Model file for the job. Use its own axes, mm. A direction names the side the tool comes from. Give positions to 0.01 mm unless a question says otherwise; leave off trailing zeros. Loops run counter-clockwise (first coordinate to the right, second up) from the corner with the lowest first, then second, coordinate; pieces in that order, holes last. Notation, with made-up numbers: (48.5, -13) -> (70.5, -13) arc R20 cw to (70.5, 20) -> close; hole circle Ø10 at (77.5, -24.5). An arc over 180 degrees is marked (long way). Use CSV: the item, a comma, the result in double quotes. Start each with the question number.
(1) Flat gauge pins, fed straight in: pin 1 (0.6 mm diameter, centred on y = 9, z = 2, fed in from +X); pin 2 (1.6 mm diameter, centred on y = 14.5, z = 1, fed in from -X); pin 3 (0.9 mm diameter, centred on y = 12, z = 2, fed in from +X). Where does each tip first touch, or does it go through?
(2) 3-axis set-ups, long thin cutter, end or side, ignore diameter. For faces 4 (the flat face through (4.255, 14, 1)), 5 (the flat face through (5, 11.124, 1)), 6 (the flat face through (2.646, 10, 1)), 7 (the flat face through (1.128, 16, -4)), 8 (the cylindrical face through (-5.7, 4.7, -2)): which of +Z, -Z, +X, -X, +Y, -Y reach the whole face in a straight line?
(3) Cut at B-B on x = -2.25. Write the cut outline in (y, z).
(4) Cut at C-C on x = 8. Write the cut outline in (y, z).
(5) Cut at A-A on y = 16. State how many separate pieces and enclosed holes the cut face has, then the cut area to 3 significant figures.
(6) Pull direction X, two halves, no side cores. Call faces 1 (the flat face through (-0.14, 22.86, 1.48)), 2 (the flat face through (-3, 10, -1)), 3 (the flat face through (3.12, 7.43, 1.48)): pulls with the +X half, pulls with the -X half, needs draft (parallel to the pull), parting line crosses it, or undercut.
(7) Cut at D-D on y = 22. Write the cut outline in (x, z), then the cut area to 3 significant figures.
(8) Drill centre lines: probe 1 along X at (y, z) = (2, -3); probe 2 along X at (y, z) = (3, -2.75); probe 3 along Z at (x, y) = (4.75, -0.5). Where is each one in solid material? Low to high.
from build123d import *

# Parameters (mm, degrees)
BOSS_SWITCH_BODY_DEPTH                    = 3
SKETCH1_W                                 = 4.0875
SKETCH1_H                                 = 1.5
SKETCH1_W_2                               = 3.046903414
SKETCH1_H_2                               = 3.5
BOSS_FLANGE_WIDTH_DEPTH                   = 5
SKETCH2_W                                 = 4
SKETCH2_H                                 = 2
SKETCH2_W_2                               = 8
SKETCH2_H_2                               = 1.5
BOSS_FLANGE_HEIGHT_DEPTH                  = 10.620596586
CUT_UP_TO_DOWN_DERAILLEUR_CLEARANCE_REACH = 23.629
SKETCH10_W                                = 1.5
SKETCH10_H                                = 3
SKETCH17_W                                = 12.1675
SKETCH17_H                                = 4
BOSS_FLANGE_SUPPORT_DEPTH                 = 17.508325141
TAP_DRILL_FOR_M2X0_4_TAP1_D               = 1.6
M2_CLEARANCE_HOLE2_D                      = 2.4
M2_CLEARANCE_HOLE2_DEPTH                  = 15
M2_CLEARANCE_HOLE2_TIP                    = 0.721032743
CHAMFER_FLANGE_SUPPORT_SIZE               = 1.5
CHAMFER_FLANGE_SUPPORT_2_SIZE             = 1.5
SKETCH23_W                                = 7.349718646
SKETCH23_H                                = 15.508325141
CUT_GAP_FOR_PRINTING_DEPTH                = 32.000499688
CUT_WIDE_DERAILLEUR_CLEARANCE_DEPTH       = 33.195879702
CUT_WIDE_DERAILLEUR_CLEARANCE_DEPTH_BACK  = 4
SKETCH27_W                                = 2.5
SKETCH27_H                                = 3.5
CHAMFER9_SIZE                             = 1.25
SKETCH28_W                                = 3.046903414
SKETCH28_H                                = 1
CUT_EXTRUDE1_DEPTH                        = 1
CHAMFER10_SIZE                            = 0.5
CHAMFER_FLANGE_SUPPORT_3_SIZE             = 1
CUT_EXTRUDE2_DEPTH                        = 34.862828732
BOSS_EXTRUDE2_DEPTH                       = 8.2


with BuildPart() as part:
    # Sketch-SwitchBossUp → Boss-Switch Body (new body)
    with BuildSketch(Plane.XY):
        with BuildLine():
            Line((5.581091204, 12.554885442), (5.58109997, 11.370542897))
            Line((5.58109997, 11.370542897), (5.154266051, 11.12411022))
            Line((5.154266051, 11.12411022), (3.971266051, 11.12411022))
            Line((3.971266051, 11.12411022), (3.97126394, 11.79911022))
            Line((3.97126394, 11.79911022), (3.296271341, 11.409403061))
            Line((3.296271341, 11.409403061), (3.296271341, 9.409403061))
            Line((3.296271341, 9.409403061), (3.971278743, 9.019687356))
            Line((3.971278743, 9.019687356), (3.971278743, 9.409408058))
            Line((3.971278743, 9.409408058), (5.333511297, 10.40941814))
            Line((5.333511297, 10.40941814), (6.133511297, 10.409424062))
            Line((6.133511297, 10.409424062), (6.627976927, 9.860264345))
            Line((6.627976927, 9.860264345), (6.627976927, 8.007577878))
            Line((6.627976927, 8.007577878), (6.081127833, 7.606137899))
            Line((6.081127833, 7.606137899), (5.581127833, 7.606137899))
            Line((5.581127833, 7.606137899), (4.906138119, 7.216432406))
            Line((4.906138119, 7.216432406), (4.906138119, 5.216432406))
            Line((4.906138119, 5.216432406), (5.58114552, 4.826716701))
            Line((5.58114552, 4.826716701), (6.290476927, 4.826716701))
            Line((6.290476927, 4.826716701), (6.290476927, 3.076720436))
            Line((6.290476927, 3.076720436), (5.040476927, 1.826720436))
            Line((5.040476927, 1.826720436), (5.040476927, -0.673279564))
            Line((5.040476927, -0.673279564), (6.627976927, -0.673279564))
            Line((6.627976927, -0.673279564), (6.627976927, -3.673279564))
            Line((6.627976927, -3.673279564), (2.540476927, -3.673279564))
            Line((2.540476927, -3.673279564), (2.540476927, -2.173279564))
            Line((2.540476927, -2.173279564), (4.040476927, -0.673279564))
            Line((4.040476927, -0.673279564), (4.040476927, 1.826720436))
            Line((4.040476927, 1.826720436), (2.790476927, 3.076720436))
            Line((2.790476927, 3.076720436), (2.790476927, 4.826720436))
            Line((2.790476927, 4.826720436), (3.58114552, 4.826720436))
            Line((3.58114552, 4.826720436), (4.256138119, 5.216427595))
            Line((4.256138119, 5.216427595), (4.256138119, 7.216427595))
            Line((4.256138119, 7.216427595), (3.581130717, 7.6061433))
            Line((3.581130717, 7.6061433), (2.64686251, 7.249572244))
            Line((2.64686251, 7.249572244), (1.971281627, 9.019692757))
            Line((1.971281627, 9.019692757), (2.646271341, 9.40939825))
            Line((2.646271341, 9.40939825), (2.646271341, 11.40939825))
            Line((2.646271341, 11.40939825), (1.696557212, 11.957715958))
            Line((1.696557212, 11.957715958), (0.573317845, 12.60621851))
            Line((0.573317845, 12.60621851), (-0.645153605, 19.844362607))
            ThreePointArc((-0.645153605, 19.844362607), (-0.473707256, 20.590279886), (0.174966786, 20.996492176))
            Line((0.174966786, 20.996492176), (-0.46073685, 24.772792819))
            ThreePointArc((-0.46073685, 24.772792819), (-1.019582136, 24.919522879), (-1.541303694, 25.167805745))
            ThreePointArc((-1.541303694, 25.167805745), (-2.872284003, 26.795385437), (-2.852546321, 28.897797067))
            ThreePointArc((-2.852546321, 28.897797067), (-1.887813913, 29.338582026), (-1.447028953, 28.373849618))
            ThreePointArc((-1.447028953, 28.373849618), (-0.703448682, 26.416936722), (1.333779254, 26.898727173))
            ThreePointArc((1.333779254, 26.898727173), (2.379722745, 27.074801628), (2.555797201, 26.028858137))
            ThreePointArc((2.555797201, 26.028858137), (2.086504637, 25.507104397), (1.511513111, 25.104801997))
            Line((1.511513111, 25.104801997), (1.553598189, 24.854801997))
            Line((1.553598189, 24.854801997), (9.027976927, 24.854801997))
            Line((9.027976927, 24.854801997), (9.027976927, 22.354801997))
            Line((9.027976927, 22.354801997), (9.027976927, 20.354801997))
            Line((9.027976927, 20.354801997), (2.311129602, 20.354801997))
            Line((2.311129602, 20.354801997), (3.620242387, 12.578216848))
            Line((3.620242387, 12.578216848), (4.255457038, 12.944958198))
            Line((4.255457038, 12.944958198), (4.255457038, 14.944958198))
            Line((4.255457038, 14.944958198), (3.579805878, 15.335045577))
            Line((3.579805878, 15.335045577), (3.581073513, 15.335045577))
            Line((3.581073513, 15.335045577), (3.581073513, 17.835045577))
            Line((3.581073513, 17.835045577), (5.725580434, 17.835045577))
            Line((5.725580434, 17.835045577), (6.627976927, 17.835045577))
            Line((6.627976927, 17.835045577), (6.627976927, 14.94496801))
            Line((6.627976927, 14.94496801), (6.081099865, 15.335045577))
            Line((6.081099865, 15.335045577), (5.581099865, 15.335045577))
            Line((5.581099865, 15.335045577), (4.905457038, 14.944963009))
            Line((4.905457038, 14.944963009), (4.905457038, 12.944963009))
            Line((4.905457038, 12.944963009), (5.581091204, 12.554885442))
        make_face()
    extrude(amount=BOSS_SWITCH_BODY_DEPTH)

    # Sketch1 → Boss-Flange Width (add)
    with BuildSketch(Plane(origin=(0, 0, 0), x_dir=(-1, 0, 0), z_dir=(0, 0, -1))):
        with Locations((-4.584226927, -2.923279564)):
            Rectangle(SKETCH1_W, SKETCH1_H)
        with Locations((-5.10452522, 17.085045577)):
            Rectangle(SKETCH1_W_2, SKETCH1_H_2)
    extrude(amount=BOSS_FLANGE_WIDTH_DEPTH)

    # Sketch2 → Boss-Flange Height (add)
    with BuildSketch(Plane(origin=(-7.039523073, 0, 0), x_dir=(0, 0, -1), z_dir=(1, 0, 0))):
        with Locations((3, 16.335045577)):
            Rectangle(SKETCH2_W, SKETCH2_H)
        with Locations((1, -2.923279564)):
            Rectangle(SKETCH2_W_2, SKETCH2_H_2)
    extrude(amount=BOSS_FLANGE_HEIGHT_DEPTH)

    # Sketch10 → Cut-Up-To-Down Derailleur Clearance (cut, up to next)
    with BuildSketch(Plane(origin=(0, 15.335045577, 0), x_dir=(1, 0, 0), z_dir=(0, 1, 0)), mode=Mode.PRIVATE) as cut_up_to_down_derailleur_clearance_sk1:
        with Locations((5.877976927, 3.5)):
            Rectangle(SKETCH10_W, SKETCH10_H)
    cut_up_to_down_derailleur_clearance_tool1 = extrude(cut_up_to_down_derailleur_clearance_sk1.sketch, amount=CUT_UP_TO_DOWN_DERAILLEUR_CLEARANCE_REACH, mode=Mode.PRIVATE) & part.part
    add(cut_up_to_down_derailleur_clearance_tool1.solids().sort_by_distance((5.877977, 15.335046, -3.5))[0], mode=Mode.SUBTRACT)

    # Sketch17 → Boss-Flange Support (add)
    with BuildSketch(Plane.XZ.offset(-15.335045577)):
        with Locations((-0.955773073, -3)):
            Rectangle(SKETCH17_W, SKETCH17_H)
    extrude(amount=BOSS_FLANGE_SUPPORT_DEPTH)

    # Tap Drill for M2x0.4 Tap1 (through all)
    with Locations(Plane(origin=(0, -3.673279564, 0), x_dir=(-1, 0, 0), z_dir=(0, -1, 0))):
        with Locations((5.039523073, 3), (0.539523073, 3)):
            Hole(TAP_DRILL_FOR_M2X0_4_TAP1_D / 2)

    # M2 Clearance Hole2
    with Locations(Plane.XZ.offset(3.673279564)):
        with Locations((-5.039523073, -3), (-0.539523073, -3)):
            Hole(M2_CLEARANCE_HOLE2_D / 2, depth=M2_CLEARANCE_HOLE2_DEPTH)
            with Locations((0, 0, -(M2_CLEARANCE_HOLE2_DEPTH + M2_CLEARANCE_HOLE2_TIP / 2))):  # 118° drill point
                Cone(0, M2_CLEARANCE_HOLE2_D / 2, M2_CLEARANCE_HOLE2_TIP, mode=Mode.SUBTRACT)

    # Chamfer-Flange Support
    chamfer_flange_support_edges = [part.edges().sort_by_distance(p)[0] for p in [
        (3.581073513, 17.335045577, -3),
    ]]
    chamfer(chamfer_flange_support_edges, length=CHAMFER_FLANGE_SUPPORT_SIZE - 0.0001)  # a hair under: the kernel refuses the full size

    # Chamfer-Flange Support 2
    chamfer_flange_support_2_edges = [part.edges().sort_by_distance(p)[0] for p in [
        (5.127976927, 17.085045577, -2),
        (5.127976927, 15.335045577, -1.5),
    ]]
    chamfer(chamfer_flange_support_2_edges, length=CHAMFER_FLANGE_SUPPORT_2_SIZE - 0.0001)  # a hair under: the kernel refuses the full size

    # Sketch23 → Cut-Gap for Printing (cut, through all)
    with BuildSketch(Plane.XY.offset(-1)):
        with Locations((4.83533625, 7.580883007)):
            Rectangle(SKETCH23_W, SKETCH23_H)
    extrude(amount=-CUT_GAP_FOR_PRINTING_DEPTH, mode=Mode.SUBTRACT)

    # Sketch27 → Cut-Wide Derailleur Clearance (cut, two sides: drawn at the far end of the back side and taken through both)
    with BuildSketch(Plane(origin=(5.127976927, 0, 0), x_dir=(0, 0, -1), z_dir=(1, 0, 0)).offset(-CUT_WIDE_DERAILLEUR_CLEARANCE_DEPTH_BACK)):
        with Locations((3.75, 17.085045577)):
            Rectangle(SKETCH27_W, SKETCH27_H)
    extrude(amount=CUT_WIDE_DERAILLEUR_CLEARANCE_DEPTH + CUT_WIDE_DERAILLEUR_CLEARANCE_DEPTH_BACK, mode=Mode.SUBTRACT)

    # Chamfer9
    chamfer9_edges = [part.edges().sort_by_distance(p)[0] for p in [
        (4.85447522, 18.835045577, -2.5),
    ]]
    chamfer(chamfer9_edges, length=CHAMFER9_SIZE)

    # Sketch28 → Cut-Extrude1 (cut)
    with BuildSketch(Plane.XY.offset(-1)):
        with Locations((5.10452522, 18.335045577)):
            Rectangle(SKETCH28_W, SKETCH28_H)
    extrude(amount=CUT_EXTRUDE1_DEPTH, mode=Mode.SUBTRACT)

    # Chamfer10
    chamfer10_edges = [part.edges().sort_by_distance(p)[0] for p in [
        (3.581073513, 16.335045577, -1),
        (5.10452522, 17.835045577, -1),
    ]]
    chamfer(chamfer10_edges, length=CHAMFER10_SIZE - 0.0001)  # a hair under: the kernel refuses the full size

    # Chamfer-Flange Support 3
    chamfer_flange_support_3_edges = [part.edges().sort_by_distance(p)[0] for p in [
        (-0.955773073, -2.173279564, -1),
    ]]
    chamfer(chamfer_flange_support_3_edges, length=CHAMFER_FLANGE_SUPPORT_3_SIZE - 0.0001)  # a hair under: the kernel refuses the full size

    # Sketch31 → Cut-Extrude2 (cut, through all)
    with BuildSketch(Plane.ZY.offset(7.039523073)):
        Polygon((-5, -2.180661432), (-5, -3.673279564), (0, -3.673279564), (-1.492618132, -2.180661432), align=None)
    extrude(amount=-CUT_EXTRUDE2_DEPTH, mode=Mode.SUBTRACT)

    # Sketch32 → Boss-Extrude2 (add)
    with BuildSketch(Plane.ZY.offset(7.039523073)):
        Polygon((3, -2.173279564), (-1, 1.826720436), (-1, -2.082793031), (0.406297605, -3.355496176), (3, -3.355496176), align=None)
    extrude(amount=-BOSS_EXTRUDE2_DEPTH)


solid = part.part
Check result:
1,pin 1,"x = 6.63"
1,pin 2,"x = 0.12"
1,pin 3,"x = 5.58"
2,face 4,"+Z, -Z"
2,face 5,"+Z, -Z, +X"
2,face 6,"+Z, -Z, -X"
2,face 7,"-Z, +X, +Y"
2,face 8,"-Y"
3,outline,"(-3.67, 0) -> (-2.18, -1.49) -> (-2.18, -5) -> (17.34, -5) -> (17.34, -1) -> (1.83, -1) -> (-2.17, 3) -> (-3.67, 3) -> close; (25.75, 0) -> (29.38, 0) -> (29.38, 3) -> (25.75, 3) -> close"
4,outline,"(20.35, 0) -> (24.85, 0) -> (24.85, 3) -> (20.35, 3) -> close"
5,separate pieces,"2"
5,enclosed holes,"2"
5,area,"58.2 mm²"
6,face 1,"pulls with the -X half"
6,face 2,"needs draft"
6,face 3,"undercut"
7,outline,"(0.01, 0) -> (9.03, 0) -> (9.03, 3) -> (0.01, 3) -> close"
7,area,"27.1 mm²"
8,probe 1,"-7.04 to -6.24, -3.84 to -1.74, 0.66 to 1.16"
8,probe 2,"-7.04 to -6.21, -3.87 to -1.71, 0.63 to 1.16"
8,probe 3,"-5 to -1, 0 to 3"
